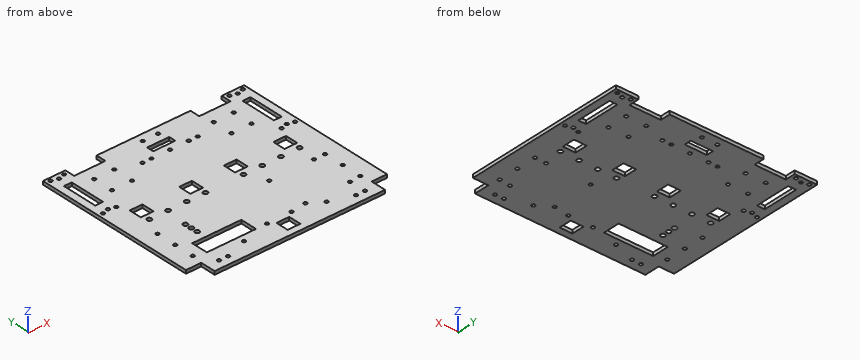
from build123d import *

# Parameters (mm, degrees)
SKETCH_R      = 1.5
SKETCH_R_2    = 2
SKETCH_W      = 7
SKETCH_H      = 32
SKETCH_W_2    = 11.4
SKETCH_H_2    = 11.4
PAD_DEPTH     = 3
SKETCH001_R   = 1.5
SKETCH001_R_2 = 2
SKETCH001_W   = 19.8
SKETCH001_H   = 6.2
SKETCH001_W_2 = 44
SKETCH001_H_2 = 15
POCKET_DEPTH  = 3.001


with BuildPart() as part:
    # Sketch → Pad (new body)
    with BuildSketch(Plane.XY):
        Polygon((90, 160), (90, 17.4), (84.3, 17.4), (84.3, 6), (90, 6), (90, 0), (13.7, 0), (13.7, 13.7), (0, 13.7), (0, 160), (20, 160), (20, 151), (48, 151), (48, 160), align=None)
        with Locations((10, 155)):
            Circle(SKETCH_R, mode=Mode.SUBTRACT)
        with Locations((10, 105)):
            Circle(SKETCH_R, mode=Mode.SUBTRACT)
        with Locations((27.5, 139.05)):
            Circle(SKETCH_R, mode=Mode.SUBTRACT)
        with Locations((45.5, 139.05)):
            Circle(SKETCH_R, mode=Mode.SUBTRACT)
        with Locations((27.5, 120.95)):
            Circle(SKETCH_R, mode=Mode.SUBTRACT)
        with Locations((45.5, 120.95)):
            Circle(SKETCH_R, mode=Mode.SUBTRACT)
        with Locations((4, 156.75)):
            Circle(SKETCH_R, mode=Mode.SUBTRACT)
        with Locations((16, 156.75)):
            Circle(SKETCH_R, mode=Mode.SUBTRACT)
        with Locations((4, 103.25)):
            Circle(SKETCH_R, mode=Mode.SUBTRACT)
        with Locations((16, 103.25)):
            Circle(SKETCH_R, mode=Mode.SUBTRACT)
        with Locations((24.7, 8)):
            Circle(SKETCH_R, mode=Mode.SUBTRACT)
        with Locations((32.7, 8)):
            Circle(SKETCH_R, mode=Mode.SUBTRACT)
        with Locations((79, 21)):
            Circle(SKETCH_R, mode=Mode.SUBTRACT)
        with Locations((22.74, 77.15)):
            Circle(SKETCH_R_2, mode=Mode.SUBTRACT)
        with Locations((39.48, 77.15)):
            Circle(SKETCH_R_2, mode=Mode.SUBTRACT)
        with Locations((56.22, 77.15)):
            Circle(SKETCH_R_2, mode=Mode.SUBTRACT)
        with Locations((72.96, 77.15)):
            Circle(SKETCH_R_2, mode=Mode.SUBTRACT)
        with Locations((53, 14.9)):
            Circle(SKETCH_R, mode=Mode.SUBTRACT)
        with Locations((15, 59.91)):
            Circle(SKETCH_R, mode=Mode.SUBTRACT)
        with Locations((15, 41.91)):
            Circle(SKETCH_R, mode=Mode.SUBTRACT)
        with Locations((15, 23.91)):
            Circle(SKETCH_R, mode=Mode.SUBTRACT)
        with Locations((10, 130)):
            Rectangle(SKETCH_W, SKETCH_H, mode=Mode.SUBTRACT)
        with Locations((25.7, 88.45)):
            Rectangle(SKETCH_W_2, SKETCH_H_2, mode=Mode.SUBTRACT)
        with Locations((70, 88.45)):
            Rectangle(SKETCH_W_2, SKETCH_H_2, mode=Mode.SUBTRACT)
    pad = extrude(amount=PAD_DEPTH)

    # Mirrored: Pad across face of Pad
    add(pad.mirror(Plane(origin=(90, 88.7, 1.5), x_dir=(0, 1, 0), z_dir=(1, 0, 0))))

    # Sketch001 → Pocket (cut, through all)
    with BuildSketch(Plane.XY.offset(3)):
        with Locations((90, 132.8)):
            Circle(SKETCH001_R)
        with Locations((106.7, 132.8)):
            Circle(SKETCH001_R)
        with Locations((114.7, 132.8)):
            Circle(SKETCH001_R)
        with Locations((73.3, 132.8)):
            Circle(SKETCH001_R)
        with Locations((65.3, 132.8)):
            Circle(SKETCH001_R)
        with Locations((96.9, 153)):
            Circle(SKETCH001_R)
        with Locations((83.1, 153)):
            Circle(SKETCH001_R)
        with Locations((37, 56.5)):
            Circle(SKETCH001_R_2)
        with Locations((37, 50.5)):
            Circle(SKETCH001_R_2)
        with Locations((37, 44.5)):
            Circle(SKETCH001_R_2)
        with Locations((115, 59.9)):
            Circle(SKETCH001_R)
        with Locations((155, 59.9)):
            Circle(SKETCH001_R)
        with Locations((115, 22.9)):
            Circle(SKETCH001_R)
        with Locations((155, 22.9)):
            Circle(SKETCH001_R)
        with Locations((90, 141.9)):
            Rectangle(SKETCH001_W, SKETCH001_H)
        with Locations((47, 28.4)):
            Rectangle(SKETCH001_W_2, SKETCH001_H_2)
    extrude(amount=-POCKET_DEPTH, mode=Mode.SUBTRACT)


solid = part.part
Verification items for the finished model (mm, model axes). Coordinates: 2 decimals unless noted, no trailing zeros. Order: outer loops, then holes, each group sorted by start corner. A loop starts at its lowest first (then second) coordinate and runs counter-clockwise, first axis right, second up. Notation, with made-up numbers: M 2.25,-31.75 L 27.25,-31.75 A24 cw 27.25,-10.75 Z; hole C -29,57.5 d9. An arc over 180 degrees is marked long. One line per item, written item: value. Start each with the question number.
Item 1: Sectioned sample at B-B (y = 116). Enter the section's corners in (x, z), then the cut area to 3 significant figures.
Item 2: Gauge pin test, flat end, axial feed: pin 1 (2.5 mm diameter, centred on x = 27.5, y = 139.05, fed in from -Z). Record the tip position at first contact, or that the pin passes through.
Item 3: Sectioned sample at D-D (z = 1.65). Count the separate pieces of the cut face and the enclosed holes in it, then the cut area to 3 significant figures.
Item 4: Sectioned sample at C-C (y = 142.5). Enter the section's corners in (x, z).
Item 5: Scan lines: probe 1 along Y at (x, z) = (83, 2.2); probe 2 along Y at (x, z) = (152.5, 2); probe 3 along Y at (x, z) = (65.3, 0.95). Record each from-to range of solid material in increasing order.
Item 6: Sectioned sample at A-A (y = 28). Enter the section's corners in (x, z).
Conclusion:
1. outline: M 0,0 L 6.5,0 L 6.5,3 L 0,3 Z; M 13.5,0 L 166.5,0 L 166.5,3 L 13.5,3 Z; M 173.5,0 L 180,0 L 180,3 L 173.5,3 Z
1. area: 498 mm^2
2. pin 1: passes through
3. separate pieces: 1
3. enclosed holes: 65
3. area: 25,600 mm^2
4. outline: M 0,0 L 6.5,0 L 6.5,3 L 0,3 Z; M 13.5,0 L 80.1,0 L 80.1,3 L 13.5,3 Z; M 99.9,0 L 166.5,0 L 166.5,3 L 99.9,3 Z; M 173.5,0 L 180,0 L 180,3 L 173.5,3 Z
5. probe 1: y = 0 to 138.8, 145 to 151.5, 154.5 to 160
5. probe 2: y = 0 to 82.75, 94.15 to 119.45, 122.45 to 137.55, 140.55 to 151
5. probe 3: y = 0 to 20.9, 35.9 to 82.75, 94.15 to 131.3, 134.3 to 160
6. outline: M 0,0 L 25,0 L 25,3 L 0,3 Z; M 69,0 L 180,0 L 180,3 L 69,3 Z
